from build123d import *

# Parameters (mm, degrees)
SKETCH2_R           = 2.5
BOSS_EXTRUDE1_DEPTH = 4
FILLET1_R           = 3
CUT_EXTRUDE2_DEPTH  = 7
FILLET2_R           = 3
FILLET3_R           = 2
CUT_EXTRUDE3_DEPTH  = 4
FILLET4_R           = 3
CUT_EXTRUDE4_DEPTH  = 5
FILLET5_R           = 3


with BuildPart() as part:
    # Sketch2 → Boss-Extrude1 (new body)
    with BuildSketch(Plane(origin=(0, 0, 0), x_dir=(1, 0, 0), z_dir=(0, 1, 0))):
        with BuildLine():
            ThreePointArc((70.082441242, 70.375471459), (68.701032678, 85.785425288), (84.157953122, 85.10824213))
            ThreePointArc((84.157953122, 85.10824213), (88.169530247, 76.167900978), (87.971523368, 85.965004847))
            ThreePointArc((87.971523368, 85.965004847), (66.773130519, 88.957801307), (67.785886209, 67.573156911))
            ThreePointArc((67.785886209, 67.573156911), (76.405902982, 62.851068524), (70.082441242, 70.375471459))
        make_face()
        with Locations(Location((72.538655529, 66.020358214, 0), (0, 0, 270))):
            Circle(SKETCH2_R, mode=Mode.SUBTRACT)
        with Locations(Location((87.073540725, 81.04630307, 0), (0, 0, 270))):
            Circle(SKETCH2_R, mode=Mode.SUBTRACT)
    extrude(amount=BOSS_EXTRUDE1_DEPTH)

    # Fillet1
    fillet1_edges = [part.edges().sort_by_distance(p)[0] for p in [
        (84.157953122, 2, -85.10824213),
        (70.082441242, 2, -70.375471459),
        (67.785886209, 2, -67.573156911),
        (87.971523368, 2, -85.965004847),
    ]]
    fillet(fillet1_edges, radius=FILLET1_R)

    # Sketch4 → Cut-Extrude2 (cut)
    with BuildSketch(Plane(origin=(0, 0, 0), x_dir=(-1, 0, 0), z_dir=(0, -1, 0))):
        Polygon((-78.063653069, 66.716653157), (-72.1449642, 71.091471725), (-73.077184563, 72.352671977), (-78.995873431, 67.977853409), align=None)
    extrude(amount=-CUT_EXTRUDE2_DEPTH, mode=Mode.SUBTRACT)

    # Fillet2
    fillet2_edges = [part.edges().sort_by_distance(p)[0] for p in [
        (77.394817884, 2, -67.211024909),
    ]]
    fillet(fillet2_edges, radius=FILLET2_R)

    # Fillet3
    fillet3_edges = [part.edges().sort_by_distance(p)[0] for p in [
        (72.252278132, 2, -71.012150275),
    ]]
    fillet(fillet3_edges, radius=FILLET3_R)

    # Sketch5 → Cut-Extrude3 (cut)
    with BuildSketch(Plane(origin=(0, 4, 0), x_dir=(1, 0, 0), z_dir=(0, 1, 0))):
        Polygon((91.915683274, 82.292760262), (87.509474915, 76.065343184), (89.248604191, 74.615528375), (94.045863103, 81.084803637), align=None)
    extrude(amount=-CUT_EXTRUDE3_DEPTH, mode=Mode.SUBTRACT)

    # Fillet4
    fillet4_edges = [part.edges().sort_by_distance(p)[0] for p in [
        (91.915683274, 2, -82.292760262),
        (87.509474915, 2, -76.065343184),
    ]]
    fillet(fillet4_edges, radius=FILLET4_R)

    # Sketch6 → Cut-Extrude4 (cut)
    with BuildSketch(Plane(origin=(0, 4, 0), x_dir=(1, 0, 0), z_dir=(0, 1, 0))):
        Polygon((88.770033289, 77.846925466), (84.083019815, 77.039211271), (84.659332186, 75.34612768), (89.090596179, 75.986759337), align=None)
    extrude(amount=-CUT_EXTRUDE4_DEPTH, mode=Mode.SUBTRACT)

    # Fillet5
    fillet5_edges = [part.edges().sort_by_distance(p)[0] for p in [
        (88.770033289, 2, -77.846925466),
        (84.083019815, 2, -77.039211271),
    ]]
    fillet(fillet5_edges, radius=FILLET5_R)


solid = part.part
Input: part model. Units: mm. Frame: model coordinates. A direction names the side the tool comes from. Give positions to 0.01 mm unless a question says otherwise; leave off trailing zeros. Write each loop counter-clockwise with the first axis right and the second up, starting at its lowest first coordinate (ties: lowest second). Pieces come first, ordered by that corner, then holes. Notation, with made-up numbers: M 35.25,62 L 41.25,62 A23 ccw 41.25,87 Z; hole C 13.25,56 d2. An arc over 180 degrees is marked long. Write item = value, one per line. Start each with the question number.
1) Cut plane A-A on x = 74.25. Return the cut outline in (y, z).
2) Draft query along X for faces 1 (the cylindrical face through (67.22, 1.97, -89.35)), 2 (the cylindrical face through (71.017, 1.972, -68.004)), 3 (the flat face through (70.3, 4, -87.4)). Return one class per face: +X half, -X half, draft (parallel to the pull), parting line (faces both ways), or undercut.
3) Reachability of faces 4 (the cylindrical face through (82.08, 1.97, -81.33)), 5 (the cylindrical face through (83.8, 1.97, -77.64)), 6 (the flat face through (74.62, 1.97, -69.26)) from +Z, -Z, +X, -X, +Y, -Y: full face, straight path, thin tool, end or side. Return the list, or none.
4) Material intervals for line 1 along Z through (x, y) = (72.5, 0.5); line 2 along Z through (x, y) = (73.5, 2.6); line 3 along X through (y, z) = (2.15, -65), sorted ascending. Write a range as [from, to].
5) Cut plane D-D on y = 0.5. Count the separate pieces of the cut face and the enclosed holes in it, then the cut area to 3 significant figures.
6) Cut plane B-B on z = -83. Return the cut outline in (x, y).
7) First-contact query: pin 1 Ø1.5 at (y, z) = (1.5, -84) entering from +X. Flat tip, straight axial feed; report the tip coordinate or a pass-through.
8) Cut plane C-C on x = 66.25. Return the cut outline in (y, z), then the cut area to 3 significant figures.
Solved:
q1.outline = M 0,-92.45 L 4,-92.45 L 4,-88.79 L 0,-88.79 Z; M 0,-69.54 L 4,-69.54 L 4,-67.84 L 0,-67.84 Z; M 0,-64.2 L 4,-64.2 L 4,-61.32 L 0,-61.32 Z
q2.face_1 = parting line
q2.face_2 = undercut
q2.face_3 = draft
q3.face_4 = +Y, -Y
q3.face_5 = +Z, +Y, -Y
q3.face_6 = +X, +Y, -Y
q4.line_1 = [-92.1, -88.3], [-70.76, -68.52], [-63.52, -61.02]
q4.line_2 = [-92.33, -88.62], [-70.09, -68.33], [-63.71, -61.11]
q4.line_3 = [67.64, 70.26], [74.82, 77.43]
q5.separate_pieces = 1
q5.enclosed_holes = 2
q5.area = 250 mm2
q6.outline = M 62.92,0 L 66.8,0 L 66.8,4 L 62.92,4 Z; M 82.47,0 L 85.51,0 L 85.51,4 L 82.47,4 Z; M 88.63,0 L 91.37,0 L 91.37,4 L 88.63,4 Z
q7.pin_1 = 91.32
q8.outline = M 0,-88.46 L 4,-88.46 L 4,-81.51 L 0,-81.51 Z; M 0,-75.86 L 4,-75.86 L 4,-68.91 L 0,-68.91 Z
q8.area = 55.6 mm2
